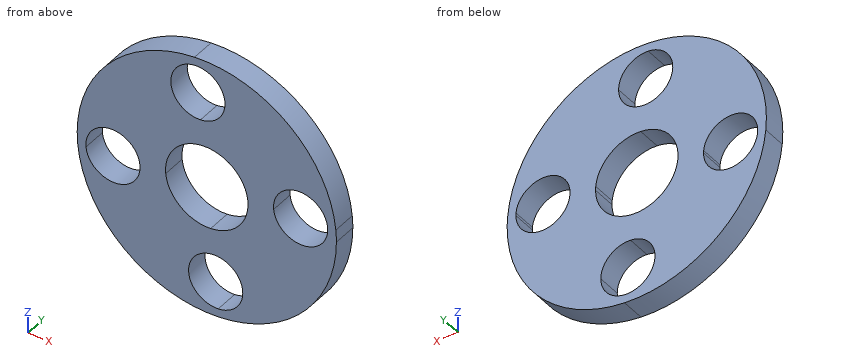
```python
from build123d import *

# Parameters (mm, degrees)
F1_DEPTH = 1


with BuildPart() as f1:
    # F0 (on Front) → F1 (new body)
    with BuildSketch(Plane.XZ):
        with BuildLine():
            ThreePointArc((-5.4755023983, -0.5185301207), (-3.5051087117, -4.2384210408), (0.5185301207, -5.4755023983))
            ThreePointArc((0.5185301207, -5.4755023983), (-1.1162060212, -4.123600864), (0.2356955176, -2.4888647257))
            ThreePointArc((0.2356955176, -2.4888647257), (-1.593231229, -1.9265550215), (-2.4888647264, -0.2356955103))
            ThreePointArc((-2.4888647264, -0.2356955103), (-2.4838547844, -0.3063252949), (-2.4821835624, -0.3771128151))
            ThreePointArc((-2.4821835624, -0.3771128151), (-3.9113960418, -1.875441593), (-5.4755023983, -0.5185301207))
        make_face()
        with BuildLine():
            ThreePointArc((-0.2356955143, 2.488864726), (-1.8704316512, 3.8407662592), (-0.5185301207, 5.4755023983))
            ThreePointArc((-0.5185301207, 5.4755023983), (-4.2384210408, 3.5051087117), (-5.4755023983, -0.5185301207))
            ThreePointArc((-5.4755023983, -0.5185301207), (-4.1236008676, 1.1162060209), (-2.4888647264, -0.2356955103))
            ThreePointArc((-2.4888647264, -0.2356955103), (-1.9265550204, 1.5932312303), (-0.2356955143, 2.488864726))
        make_face()
        with BuildLine():
            ThreePointArc((2.4888647264, 0.2356955103), (3.8407662572, 1.870431651), (5.4755023983, 0.5185301207))
            ThreePointArc((5.4755023983, 0.5185301207), (3.5051087117, 4.2384210408), (-0.5185301207, 5.4755023983))
            ThreePointArc((-0.5185301207, 5.4755023983), (0.6323112885, 5.0917163376), (1.1228871849, 3.9821835624))
            ThreePointArc((1.1228871849, 3.9821835624), (0.7324199585, 2.9727594571), (-0.2356955143, 2.488864726))
            ThreePointArc((-0.2356955143, 2.488864726), (1.5932312303, 1.9265550204), (2.4888647264, 0.2356955103))
        make_face()
        with BuildLine():
            ThreePointArc((0.5185301207, -5.4755023983), (4.0682868424, -3.7012217129), (5.5, 0))
            ThreePointArc((5.5, 0), (5.4938721859, 0.2595542422), (5.4755023983, 0.5185301207))
            ThreePointArc((5.4755023983, 0.5185301207), (5.4805123404, 0.4479003357), (5.4821835624, 0.3771128151))
            ThreePointArc((5.4821835624, 0.3771128151), (4.0529710825, -1.1212159629), (2.4888647264, 0.2356955103))
            ThreePointArc((2.4888647264, 0.2356955103), (2.4972146299, 0.1179792015), (2.5, 0))
            ThreePointArc((2.5, 0), (1.8492212948, -1.6823735028), (0.2356955176, -2.4888647257))
            ThreePointArc((0.2356955176, -2.4888647257), (1.3865369216, -2.87265079), (1.8771128151, -3.9821835624))
            ThreePointArc((1.8771128151, -3.9821835624), (1.4866455903, -4.9916076659), (0.5185301207, -5.4755023983))
        make_face()
        with BuildLine():
            Line((-5.1270613366, -0.4855327494), (-5.4755023983, -0.5185301207))
            ThreePointArc((-5.4755023983, -0.5185301207), (-3.9113960418, -1.875441593), (-2.4821835624, -0.3771128151))
            ThreePointArc((-2.4821835624, -0.3771128151), (-2.4838547844, -0.3063252949), (-2.4888647264, -0.2356955103))
            Line((-2.4888647265, -0.2356955094), (-2.8373057882, -0.2686928807))
            ThreePointArc((-2.8373057882, -0.2686928807), (-2.8334648326, -0.3228423826), (-2.8321835624, -0.3771128151))
            ThreePointArc((-2.8321835624, -0.3771128151), (-3.9279131299, -1.5258315448), (-5.1270613366, -0.4855327494))
        make_face()
        with BuildLine():
            ThreePointArc((-2.4888647264, -0.2356955103), (-4.1236008676, 1.1162060209), (-5.4755023983, -0.5185301207))
            Line((-5.4755023983, -0.5185301207), (-5.1270613366, -0.4855327494))
            ThreePointArc((-5.1270613366, -0.4855327494), (-4.0906034967, 0.7677649591), (-2.8373057882, -0.2686928807))
            Line((-2.8373057882, -0.2686928807), (-2.4888647265, -0.2356955094))
        make_face()
        with BuildLine():
            Line((-0.4855327494, 5.1270613366), (-0.5185301207, 5.4755023983))
            ThreePointArc((-0.5185301207, 5.4755023983), (-1.8704316512, 3.8407662592), (-0.2356955143, 2.488864726))
            Line((-0.2356955094, 2.4888647265), (-0.2686928807, 2.8373057882))
            ThreePointArc((-0.2686928807, 2.8373057882), (-1.5219905893, 3.8737636281), (-0.4855327494, 5.1270613366))
        make_face()
        with BuildLine():
            ThreePointArc((1.1228871849, 3.9821835624), (0.6323112885, 5.0917163376), (-0.5185301207, 5.4755023983))
            Line((-0.5185301207, 5.4755023983), (-0.4855327494, 5.1270613366))
            ThreePointArc((-0.4855327494, 5.1270613366), (0.3967789976, 4.8328253567), (0.7728871849, 3.9821835624))
            ThreePointArc((0.7728871849, 3.9821835624), (0.4735289793, 3.2082917497), (-0.2686928807, 2.8373057882))
            Line((-0.2686928807, 2.8373057882), (-0.2356955094, 2.4888647265))
            ThreePointArc((-0.2356955143, 2.488864726), (0.7324199585, 2.9727594571), (1.1228871849, 3.9821835624))
        make_face()
        with BuildLine():
            Line((0.4855327494, -5.1270613366), (0.5185301207, -5.4755023983))
            ThreePointArc((0.5185301207, -5.4755023983), (1.4866455903, -4.9916076659), (1.8771128151, -3.9821835624))
            ThreePointArc((1.8771128151, -3.9821835624), (1.3865369216, -2.87265079), (0.2356955176, -2.4888647257))
            Line((0.2356955094, -2.4888647265), (0.2686928807, -2.8373057882))
            ThreePointArc((0.2686928807, -2.8373057882), (1.1510046278, -3.1315417681), (1.5271128151, -3.9821835624))
            ThreePointArc((1.5271128151, -3.9821835624), (1.2277546094, -4.7560753751), (0.4855327494, -5.1270613366))
        make_face()
        with BuildLine():
            ThreePointArc((0.2356955176, -2.4888647257), (-1.1162060212, -4.123600864), (0.5185301207, -5.4755023983))
            Line((0.5185301207, -5.4755023983), (0.4855327494, -5.1270613366))
            ThreePointArc((0.4855327494, -5.1270613366), (-0.7677649591, -4.0906034967), (0.2686928807, -2.8373057882))
            Line((0.2686928807, -2.8373057882), (0.2356955094, -2.4888647265))
        make_face()
        with BuildLine():
            ThreePointArc((5.4821835624, 0.3771128151), (5.4805123404, 0.4479003357), (5.4755023983, 0.5185301207))
            Line((5.4755023983, 0.5185301207), (5.1270613366, 0.4855327494))
            ThreePointArc((5.1270613366, 0.4855327494), (5.1309022922, 0.4313832475), (5.1321835624, 0.3771128151))
            ThreePointArc((5.1321835624, 0.3771128151), (4.0364539949, -0.7716059147), (2.8373057882, 0.2686928807))
            Line((2.8373057882, 0.2686928807), (2.4888647265, 0.2356955094))
            ThreePointArc((2.4888647264, 0.2356955103), (4.0529710825, -1.1212159629), (5.4821835624, 0.3771128151))
        make_face()
        with BuildLine():
            Line((5.1270613366, 0.4855327494), (5.4755023983, 0.5185301207))
            ThreePointArc((5.4755023983, 0.5185301207), (3.8407662572, 1.870431651), (2.4888647264, 0.2356955103))
            Line((2.4888647265, 0.2356955094), (2.8373057882, 0.2686928807))
            ThreePointArc((2.8373057882, 0.2686928807), (3.8737636281, 1.5219905893), (5.1270613366, 0.4855327494))
        make_face()
        with BuildLine():
            Line((-0.1649868566, 1.7422053086), (-0.2356955094, 2.4888647265))
            ThreePointArc((-0.2356955143, 2.488864726), (-1.9265550204, 1.5932312303), (-2.4888647264, -0.2356955103))
            Line((-2.4888647265, -0.2356955094), (-1.7422053086, -0.1649868566))
            ThreePointArc((-1.7422053086, -0.1649868566), (-1.348588513, 1.1152618628), (-0.1649868566, 1.7422053086))
        make_face()
        with BuildLine():
            Line((1.7422053086, 0.1649868566), (2.4888647265, 0.2356955094))
            ThreePointArc((2.4888647264, 0.2356955103), (1.5932312303, 1.9265550204), (-0.2356955143, 2.488864726))
            Line((-0.2356955094, 2.4888647265), (-0.1649868566, 1.7422053086))
            ThreePointArc((-0.1649868566, 1.7422053086), (1.1152618628, 1.348588513), (1.7422053086, 0.1649868566))
        make_face()
        with BuildLine():
            ThreePointArc((-2.4888647264, -0.2356955103), (-1.593231229, -1.9265550215), (0.2356955176, -2.4888647257))
            Line((0.2356955094, -2.4888647265), (0.1649868566, -1.7422053086))
            ThreePointArc((0.1649868566, -1.7422053086), (-1.1152618628, -1.348588513), (-1.7422053086, -0.1649868566))
            Line((-1.7422053086, -0.1649868566), (-2.4888647265, -0.2356955094))
        make_face()
        with BuildLine():
            ThreePointArc((2.5, 0), (2.4972146299, 0.1179792015), (2.4888647264, 0.2356955103))
            Line((2.4888647265, 0.2356955094), (1.7422053086, 0.1649868566))
            ThreePointArc((1.7422053086, 0.1649868566), (1.748050241, 0.0825854407), (1.75, 0))
            ThreePointArc((1.75, 0), (1.2944549044, -1.1776614541), (0.1649868566, -1.7422053086))
            Line((0.1649868566, -1.7422053086), (0.2356955094, -2.4888647265))
            ThreePointArc((0.2356955176, -2.4888647257), (1.8492212948, -1.6823735028), (2.5, 0))
        make_face()
    extrude(amount=F1_DEPTH)


solid = f1.part
```
Design review of the part built by this model. Coordinates are the model's own, in mm. Round coordinates to 2 decimals unless told otherwise and drop trailing zeros. Write each loop counter-clockwise with the first axis right and the second up, starting at its lowest first coordinate (ties: lowest second). Pieces come first, ordered by that corner, then holes.
Item 1: We need section B-B on z = 4.75. Write out the cut boundary in (x, y), and give its area (3 significant figures).
Item 2: Clearance check with a flat-ended pin moving along its axis: pin 1 Ø2 at (x, z) = (-4.5, -1) entering from -Y. State where the tip first meets the part, or that it passes through.
Item 3: For probe 1 along X at (y, z) = (-0.95, -1); probe 2 along X at (y, z) = (-0.1, 1.25), list the stretches that pass through material, from the lowest coordinate up.
Item 4: We need section D-D on x = 2. Write out the cut boundary in (y, z), and give its area (3 significant figures).
Item 5: We need section C-C on x = 5. Write out the cut boundary in (y, z), and give its area (3 significant figures).
Item 6: We need section A-A on y = -0.35. Write out the cut boundary in (x, z), and give its area (3 significant figures).
Returned:
1. outline: (-2.77, -1) - (-1.23, -1) - (-1.23, 0) - (-2.77, 0) - close; (0.48, -1) - (2.77, -1) - (2.77, 0) - (0.48, 0) - close
1. area: 3.83 mm2
2. pin 1: stops at y = -1
3. probe 1: x = -5.41 to -4.95, -3.02 to -1.44, 1.44 to 5.41
3. probe 2: x = -5.36 to -1.22, 1.22 to 3.23, 4.73 to 5.36
4. outline: (-1, -5.12) - (0, -5.12) - (0, 5.12) - (-1, 5.12) - close
4. area: 10.2 mm2
5. outline: (-1, -2.29) - (0, -2.29) - (0, -0.16) - (-1, -0.16) - close; (-1, 0.91) - (0, 0.91) - (0, 2.29) - (-1, 2.29) - close
5. area: 3.51 mm2
6. outline: circle Ø11 at (0, 0); hole circle Ø2.3 at (-3.98, -0.38); hole circle Ø3.5 at (0, 0); hole circle Ø2.3 at (-0.38, 3.98); hole circle Ø2.3 at (0.38, -3.98); hole circle Ø2.3 at (3.98, 0.38)
6. area: 68.8 mm2
